Read the model definition and answer for the solid it produces. Units are mm, in the model's axes. Face numbers are marked on the shaded views. A direction names the side the tool comes from. Coordinates: 2 decimals unless noted, no trailing zeros. Order: outer loops, then holes, each group sorted by start corner. A loop starts at its lowest first (then second) coordinate and runs counter-clockwise, first axis right, second up. Notation, with made-up numbers: (-16.5, -16.75) - (42.5, -16.75) arc R14 cw to (42.5, -3.75) - close; hole circle Ø9 at (-15, 67.25). An arc over 180 degrees is marked (long way). Use one line per item in the form item = value.
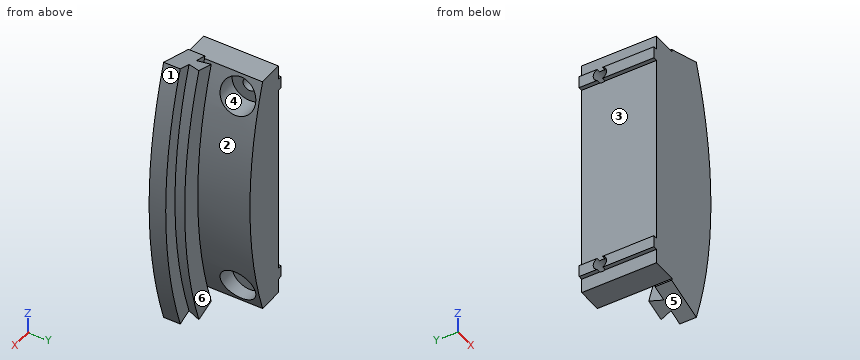
```python
from build123d import *

# Parameters (mm, degrees)
MAIN_ANGLE             = 37.5
SUPPORT_DEPTH          = 18
SKETCH6_W              = 1
SKETCH6_H              = 2.9
MAKERBEAMSUPPORT_DEPTH = 18
SKETCH7_R              = 1.6
HOLESMAKERBEAM_DEPTH   = 22.861218113
SKETCH8_R              = 4.25
CUT_EXTRUDE1_DEPTH     = 7


with BuildPart() as part:
    # Sketch1 → Main (revolve, symmetric)
    with BuildSketch(Plane.XY) as main_sk:
        Polygon((105, 0), (105, 4), (101.45, 4), (102.5, 7), (97.5, 7), (98.55, 4), (95, 4), (95, 0), align=None)
    revolve(axis=Axis((0, -0.284703924, 0), (0, 1, 0)), revolution_arc=MAIN_ANGLE / 2)
    revolve(main_sk.sketch, axis=Axis((0, -0.284703924, 0), (0, -1, 0)), revolution_arc=MAIN_ANGLE / 2)

    # Sketch2 → Support (add)
    with BuildSketch(Plane(origin=(0, 0, 0), x_dir=(-1, 0, 0), z_dir=(0, -1, 0))):
        with BuildLine():
            Line((-90.138781887, -30), (-84.138781887, -30))
            Line((-84.138781887, -30), (-84.138781887, 30))
            Line((-84.138781887, 30), (-90.138781887, 30))
            ThreePointArc((-90.138781887, 30), (-95, 0), (-90.138781887, -30))
        make_face()
    extrude(amount=-SUPPORT_DEPTH)

    # Sketch6 → MakerBeamSupport (add)
    with BuildSketch(Plane(origin=(0, 0, 0), x_dir=(1, 0, 0), z_dir=(0, 1, 0))):
        with Locations((83.638781887, -25)):
            Rectangle(SKETCH6_W, SKETCH6_H)
        with Locations((83.638781887, 25)):
            Rectangle(SKETCH6_W, SKETCH6_H)
    extrude(amount=MAKERBEAMSUPPORT_DEPTH)

    # Sketch7 → HolesMakerBeam (cut, through all)
    with BuildSketch(Plane(origin=(83.138781887, 0, 0), x_dir=(0, 0, -1), z_dir=(1, 0, 0))):
        with Locations((-25, 13)):
            Circle(SKETCH7_R)
        with Locations((25, 13)):
            Circle(SKETCH7_R)
    extrude(amount=HOLESMAKERBEAM_DEPTH, mode=Mode.SUBTRACT)

    # Sketch8 → Cut-Extrude1 (cut)
    with BuildSketch(Plane.ZY.offset(-87.138781887)):
        with Locations((25, 13)):
            Circle(SKETCH8_R)
        with Locations((-25, 13)):
            Circle(SKETCH8_R)
    extrude(amount=-CUT_EXTRUDE1_DEPTH, mode=Mode.SUBTRACT)


solid = part.part
```
(1) Section D-D, the plane y = 1.75 is taken. Write down the section's boundary in (x, z), then the cut area to 3 significant figures.
Answer list:
outline = (83.14, -26.45) - (84.14, -26.45) - (84.14, -30) - (90.14, -30) arc R95 cw to (89.96, -30.54) - (99.43, -33.75) arc R105 ccw to (99.43, 33.75) - (89.96, 30.54) arc R95 cw to (90.14, 30) - (84.14, 30) - (84.14, 26.45) - (83.14, 26.45) - (83.14, 23.55) - (84.14, 23.55) - (84.14, -23.55) - (83.14, -23.55) - close
area = 1,220 mm2
(2) Section C-C, the plane y = 13 is taken. Write down the section's boundary in (x, z), then the cut area to 3 significant figures.
Answer list:
outline = (84.14, -30) - (90.14, -30) arc R95 ccw to (90.38, -29.25) - (87.14, -29.25) - (87.14, -26.6) - (84.14, -26.6) - close; (84.14, -23.4) - (87.14, -23.4) - (87.14, -20.75) - (92.71, -20.75) arc R95 ccw to (92.71, 20.75) - (87.14, 20.75) - (87.14, 23.4) - (84.14, 23.4) - close; (84.14, 26.6) - (87.14, 26.6) - (87.14, 29.25) - (90.38, 29.25) arc R95 ccw to (90.14, 30) - (84.14, 30) - close
area = 460 mm2
(3) The mould has two halves that part along Z. Classify the marked faces 4, 5 and 6: +Z half, -Z half, draft (parallel to the pull), parting line (faces both ways), or undercut.
Answer list:
face_4 = undercut
face_5 = -Z half
face_6 = draft
(4) Straight lines are drawn through the part: L1, parallel to Z at x = 88.65, y = 13; L2, parallel to Z at x = 85.05, y = 13; L3, parallel to Y at x = 86, z = -25. For each, find the intervals that lie inside material, in ascending order.
Answer list:
L1 = -30 to -29.25, -20.75 to 20.75, 29.25 to 30
L2 = -30 to -26.6, -23.4 to 23.4, 26.6 to 30
L3 = 0 to 11.4, 14.6 to 18
(5) Section A-A, the plane y = 6 is taken. Write down the section's boundary in (x, z).
Answer list:
outline = (83.14, -26.45) - (84.14, -26.45) - (84.14, -30) - (90.14, -30) arc R95 ccw to (90.14, 30) - (84.14, 30) - (84.14, 26.45) - (83.14, 26.45) - (83.14, 23.55) - (84.14, 23.55) - (84.14, -23.55) - (83.14, -23.55) - close; (92.66, -31.45) - (96.73, -32.84) arc R102.15 ccw to (96.73, 32.84) - (92.66, 31.45) arc R97.85 cw to start
(6) Which of the six approach directions +Z, -Z, +X, -X, +Y, -Y give full straight-line access (tool end or side, diameter ignored) to the marked faces 1, 2 and 3?
Answer list:
face_1 = +X, +Y, -Y
face_2 = +Y
face_3 = -X, +Y, -Y
(7) Given pin 1 Ø7 at (y, z) = (13, 25) entering from -X; pin 2 Ø5.5 at (y, z) = (10.5, -4.5) entering from -X; pin 3 Ø1.8 at (x, y) = (86, 11.5) entering from -Z; pin 4 Ø10 at (x, z) = (101, 9) entering from +Y, each flat-ended and moving along its own axis, determine where each tip first touches the part or whether it passes through.
Answer list:
pin_1 = 83.14
pin_2 = 84.14
pin_3 = -30
pin_4 = 7
(8) Section B-B, the plane x = 85.75 is taken. Write down the section's boundary in (y, z), then the cut area to 3 significant figures.
Answer list:
outline = (0, -30) - (18, -30) - (18, 30) - (0, 30) - close; hole circle Ø3.2 at (13, -25); hole circle Ø3.2 at (13, 25)
area = 1,060 mm2
